```python
from build123d import *

# Parameters (mm, degrees)
CUT_EXTRUDE_1_DEPTH      = 14.752272539
CUT_EXTRUDE_1_DEPTH_BACK = 14.752272539
CUT_EXTRUDE_2_DEPTH      = 1.8


with BuildPart() as part:
    # Эскиз1 → Revolve 663 (revolve)
    with BuildSketch(Plane.XY, mode=Mode.PRIVATE) as revolve_663_sk:
        with BuildLine():
            Line((0, 4.75), (0, 3))
            ThreePointArc((0, 3), (0.146446609, 2.646446609), (0.5, 2.5))
            Line((0.5, 2.5), (11, 2.5))
            Line((11, 2.5), (12, 1.5))
            Line((12, 1.5), (12, 0))
            Line((12, 0), (-3.3, 0))
            ThreePointArc((-3.3, 0), (-2.645098129, 2.677305593), (-0.828287848, 4.75))
            Line((-0.828287848, 4.75), (0, 4.75))
        make_face()
    revolve(revolve_663_sk.sketch.rotate(Axis((-6.611599553, 0, 0), (1, 0, 0)), 90), axis=Axis((-6.611599553, 0, 0), (1, 0, 0)))

    # Эскиз2 → Вырез-Вытянуть1 (cut, two sides: drawn at the far end of the back side and taken through both)
    with BuildSketch(Plane.XY.offset(-CUT_EXTRUDE_1_DEPTH_BACK)):
        Polygon((-2.75, 45.30562747), (-2.75, 2.465258607), (-2.75, -2.465258607), (-2.75, -45.30562747), (-88.430737726, -45.30562747), (-88.430737726, 45.30562747), align=None)
    extrude(amount=CUT_EXTRUDE_1_DEPTH + CUT_EXTRUDE_1_DEPTH_BACK, mode=Mode.SUBTRACT)

    # Эскиз3 → Вырез-Вытянуть2 (cut)
    with BuildSketch(Plane.ZY.offset(2.75)):
        Polygon((-1.732050808, 0), (-0.866025404, -1.5), (0.866025404, -1.5), (1.732050808, 0), (0.866025404, 1.5), (-0.866025404, 1.5), align=None)
    extrude(amount=-CUT_EXTRUDE_2_DEPTH, mode=Mode.SUBTRACT)


solid = part.part
```
The model under review builds one solid part; all positions refer to its coordinate system, in mm. A direction names the side the tool comes from. Round coordinates to 2 decimals unless told otherwise and drop trailing zeros. Write each loop counter-clockwise with the first axis right and the second up, starting at its lowest first coordinate (ties: lowest second). Pieces come first, ordered by that corner, then holes.
(1) Mouldability with a two-part tool opening along Y and no side actions: class faces 1 (the flat face through (-2, 1.5, 0)), 2 (the flat face through (-2.75, 2, 0)), 3 (the cylindrical face through (-0.408, 4.637, -1.03)) as +Y half, -Y half, draft (parallel to the pull), parting line (faces both ways), or undercut.
(2) Machinability: for faces 4 (the flat face through (12, 0, 0)), 5 (the flat face through (-1.863, -0.74, -1.305)), 6 (the flat face through (0, 1, 3)), which of the approach directions +Z, -Z, +X, -X, +Y, -Y give a long, thin tool a straight path to every point of the face, cutting with its end or side? Answer none if there is none.
(3) Wall thickness on L1, parallel to Y at x = 9.5, z = 0; L2, parallel to Y at x = -1.5, z = 0; L3, parallel to Y at x = -1, z = 0.5: over which ranges is each line inside the solid? List them lowest first.
(4) We need section B-B on x = -1.25. Give the boundary of the cut face in (y, z).
(5) We need section C-C on x = 10.5. Give the boundary of the cut face in (y, z).
(6) Insertion check: pin 1 (1.5 mm diameter, centred on x = 9, y = -1.5, fed in from +Z); pin 2 (2 mm diameter, centred on y = 3, z = 3.5, fed in from +X); pin 3 (1 mm diameter, centred on y = 2.5, z = 0, fed in from +X). Each pin has a flat end and moves straight along its axis. Give the tip position at first contact, or say it passes through.
(7) We need section A-A on z = 0. Give the boundary of the cut face in (x, y).
Findings below:
1. face 1: undercut
1. face 2: draft
1. face 3: parting line
2. face 4: +Z, -Z, +X, +Y, -Y
2. face 5: -X
2. face 6: +X
3. L1: y = -2.5 to 2.5
3. L2: y = -4.2 to -1.5, 1.5 to 4.2
3. L3: y = -4.6 to -1.5, 1.5 to 4.6
4. outline: circle Ø8.85 at (0, 0); hole (-1.5, -0.87) - (0, -1.73) - (1.5, -0.87) - (1.5, 0.87) - (0, 1.73) - (-1.5, 0.87) - close
5. outline: circle Ø5 at (0, 0)
6. pin 1: stops at z = 2.38
6. pin 2: stops at x = 0
6. pin 3: stops at x = 11.5
7. outline: (-2.75, -2.47) arc R5.8 ccw to (-0.83, -4.75) - (0, -4.75) - (0, -3) arc R0.5 cw to (0.5, -2.5) - (11, -2.5) - (12, -1.5) - (12, 1.5) - (11, 2.5) - (0.5, 2.5) arc R0.5 cw to (0, 3) - (0, 4.75) - (-0.83, 4.75) arc R5.8 ccw to (-2.75, 2.47) - (-2.75, 1.5) - (-0.95, 1.5) - (-0.95, -1.5) - (-2.75, -1.5) - close
